Geometry check sheet. Reference: the model listing, model coordinates, mm. A direction names the side the tool comes from. Round coordinates to 2 decimals unless told otherwise and drop trailing zeros. Loops run counter-clockwise (first coordinate to the right, second up) from the corner with the lowest first, then second, coordinate; pieces in that order, holes last. Notation, with made-up numbers: (24.25, 63) -> (59.25, 63) arc R18 ccw to (59.25, 73) -> close; hole circle Ø7 at (-1.75, 58). An arc over 180 degrees is marked (long way). Use a Markdown table: item, result. Add a question column.
Q1. Material ranges on L1, parallel to Y at x = -9.5, z = 5.5; L2, parallel to X at y = -26, z = 0; L3, parallel to Y at x = -2, z = -2.5, recorded low to high.
Q2. Set-up check for faces 1 (the face through (-1.778, -1, 13)), 2 (the face through (3.36, -11.55, -10.66)), 3 (the face through (-0.104, -30.683, 5.601)): record each of +Z, -Z, +X, -X, +Y, -Y from which the full face is reachable in a straight line by a thin tool's end or side.
Q3. Sectioned sample at B-B, the plane y = 30.5. Enter the section's corners in (x, z).
Q4. Gauge pin test, flat ends, axial feed: P1, Ø2.5, axis at y = -27, z = 4, coming from the +X side; P2, Ø2, axis at y = 6.5, z = 15.5, coming from the +X side; P3, Ø2, axis at y = 16.5, z = -6.5, coming from the +X side; P4, Ø5.5, axis at x = -1, z = -1.5, coming from the -Y side. Record the tip position at first contact, or that the pin passes through.
Q5. Sectioned sample at A-A, the plane y = -5.5. Enter the section's corners in (x, z), then the cut area to 3 significant figures.
Q6. Release check for a two-part mould opening along Z. For faces 4 (the face through (5, -29.896, 0)), 5 (the face through (0, -28, -3.848)), 6 (the face through (7.455, -28, 2)), 7 (the face through (0, -26, 7.404)) record: released by +Z, released by -Z, zero draft, split by the parting line, or undercut.
```python
from build123d import *

# Parameters (mm, degrees)
SKETCH2_R           = 11.176
BOSS_EXTRUDE1_DEPTH = 23.4188
SKETCH3_W           = 14.9098
SKETCH3_H           = 11.2522
BOSS_EXTRUDE2_DEPTH = 9.017
SKETCH4_W           = 4.842933334
SKETCH4_H           = 7.423880536
CUT_EXTRUDE1_DEPTH  = 2.54
SKETCH5_W           = 4.779433333
SKETCH5_H           = 7.423880536
CUT_EXTRUDE2_DEPTH  = 2.54
SKETCH6_W           = 4.761113869
SKETCH6_H           = 7.423880536
CUT_EXTRUDE3_DEPTH  = 2.54
RIB1_START          = -1.778
RIB1_OUTLINE_W      = 3.294408818
RIB1_OUTLINE_H      = 2.1844
RIB1_DEPTH          = 3.556
CHAMFER1_SIZE       = 3.556
FILLET1_R           = 6.35


# Read off the part's stored shape, not the designer's step: Rib1
with BuildPart() as part:
    # Sketch1 → Revolve1 (revolve)
    with BuildSketch(Plane(origin=(0, 0, 0), x_dir=(-1, 0, 0), z_dir=(0, 0, -1)), mode=Mode.PRIVATE) as revolve1_sk:
        Polygon((-22.479, 0), (0, 0), (0, 41.1988), (-14.986000072, 41.1988), (-22.479, 21.996399801), align=None)
    revolve(revolve1_sk.sketch.rotate(Axis((0, 0, 0), (0, 1, 0)), 270), axis=Axis((0, 0, 0), (0, 1, 0)))

    # Sketch2 → Boss-Extrude1 (add)
    with BuildSketch(Plane.XZ):
        with Locations(Location((0, 0, 0), (0, 0, 270))):
            Circle(SKETCH2_R)
    extrude(amount=BOSS_EXTRUDE1_DEPTH)

    # Sketch3 → Boss-Extrude2 (add)
    with BuildSketch(Plane.XZ.offset(23.4188)):
        with Locations((0, 1.778)):
            Rectangle(SKETCH3_W, SKETCH3_H)
    extrude(amount=BOSS_EXTRUDE2_DEPTH)

    # Sketch4 → Cut-Extrude1 (cut)
    with BuildSketch(Plane.XZ.offset(32.4358)):
        Rectangle(SKETCH4_W, SKETCH4_H)
    extrude(amount=-CUT_EXTRUDE1_DEPTH, mode=Mode.SUBTRACT)

    # Sketch5 → Cut-Extrude2 (cut)
    with BuildSketch(Plane.XZ.offset(32.4358)):
        with Locations((-4.938183334, 0)):
            Rectangle(SKETCH5_W, SKETCH5_H)
    extrude(amount=-CUT_EXTRUDE2_DEPTH, mode=Mode.SUBTRACT)

    # Sketch6 → Cut-Extrude3 (cut)
    with BuildSketch(Plane.XZ.offset(32.4358)):
        with Locations((4.929023601, 0)):
            Rectangle(SKETCH6_W, SKETCH6_H)
    extrude(amount=-CUT_EXTRUDE3_DEPTH, mode=Mode.SUBTRACT)

    # Rib1 outline → Rib1 (add)
    with BuildSketch(Plane(origin=(0, 0, 0), x_dir=(0, 0, -1), z_dir=(1, 0, 0)).offset(RIB1_START)):
        with Locations((-12.647204409, -1.0922)):
            Rectangle(RIB1_OUTLINE_W, RIB1_OUTLINE_H)
    extrude(amount=RIB1_DEPTH)

    # Chamfer1
    chamfer1_edges = [part.edges().sort_by_distance(p)[0] for p in [
        (0, -32.4358, 7.4041),
    ]]
    chamfer(chamfer1_edges, length=CHAMFER1_SIZE)

    # Fillet1
    fillet1_edges = [part.edges().sort_by_distance(p)[0] for p in [
        (0, 21.996399801, -22.479),
        (0, 41.1988, -14.986000072),
        (0, 0, -22.479),
    ]]
    fillet(fillet1_edges, radius=FILLET1_R)


solid = part.part
```
Values:
| question | item | result |
|---|---|---|
| 1 | L1 | -23.42 to 41.19 |
| 1 | L2 | -7.45 to 7.45 |
| 1 | L3 | -29.9 to 41.2 |
| 2 | face 1 | +Z, -X, -Y |
| 2 | face 2 | -Y |
| 2 | face 3 | +Z, +X, -X, -Y |
| 3 | outline | circle Ø38.32 at (0, 0) |
| 4 | P1 | x = 7.45 |
| 4 | P2 | x = 17.18 |
| 4 | P3 | x = 21.8 |
| 4 | P4 | y = -32.44 |
| 5 | outline | circle Ø22.35 at (0, 0) |
| 5 | area | 392 mm^2 |
| 6 | face 4 | undercut |
| 6 | face 5 | released by -Z |
| 6 | face 6 | zero draft |
| 6 | face 7 | released by +Z |
